```python
from build123d import *

# Parameters (mm, degrees)
SKETCH1_W           = 83
SKETCH1_H           = 126.35
SKETCH1_W_2         = 57.38
SKETCH1_H_2         = 90.25
BOSS_EXTRUDE1_DEPTH = 2
SKETCH2_W           = 78.4
SKETCH2_H           = 121.75
SKETCH2_W_2         = 76.4
SKETCH2_H_2         = 119.75
BOSS_EXTRUDE2_DEPTH = 1.5
FILLET1_R           = 3


with BuildPart() as part:
    # Sketch1 → Boss-Extrude1 (new body)
    with BuildSketch(Plane(origin=(0, 0, 0), x_dir=(1, 0, 0), z_dir=(0, 1, 0))):
        Rectangle(SKETCH1_W, SKETCH1_H)
        with Locations((0, 10.75)):
            Rectangle(SKETCH1_W_2, SKETCH1_H_2, mode=Mode.SUBTRACT)
    extrude(amount=BOSS_EXTRUDE1_DEPTH)

    # Sketch2 → Boss-Extrude2 (add)
    with BuildSketch(Plane(origin=(0, 2, 0), x_dir=(1, 0, 0), z_dir=(0, 1, 0))):
        Rectangle(SKETCH2_W, SKETCH2_H)
        Rectangle(SKETCH2_W_2, SKETCH2_H_2, mode=Mode.SUBTRACT)
    extrude(amount=BOSS_EXTRUDE2_DEPTH)

    # Fillet1
    fillet1_edges = [part.edges().sort_by_distance(p)[0] for p in [
        (-41.5, 1, -63.175),
        (41.5, 1, -63.175),
        (41.5, 1, 63.175),
        (-41.5, 1, 63.175),
    ]]
    fillet(fillet1_edges, radius=FILLET1_R)


solid = part.part
```
For this review, take the finished solid that the model builds, in its own axes (mm). Round coordinates to 2 decimals unless told otherwise and drop trailing zeros. Write each loop counter-clockwise with the first axis right and the second up, starting at its lowest first coordinate (ties: lowest second). Pieces come first, ordered by that corner, then holes. Notation, with made-up numbers: (-10.5, -40) -> (-6.5, -40) arc R23 ccw to (-6.5, -17) -> close; hole circle Ø3 at (12, 2.25). An arc over 180 degrees is marked (long way). Use one line per item in the form item = value.
1) Clearance check with flat-ended pins moving along their axes: pin 1 (8 mm diameter, centred on x = 25.5, z = 35.5, fed in from +Y); pin 2 (0.8 mm diameter, centred on x = -12.5, y = 2.5, fed in from +Z) (3 decimals); pin 3 (0.8 mm diameter, centred on y = 2.5, z = 16.5, fed in from +X). State where each tip first meets the part, or that it passes through.
Found:
pin_1 = 2
pin_2 = 60.875
pin_3 = 39.2
2) Take a section at A-A, the plane z = 23. Write out the cut boundary in (x, y), and give its area (3 significant figures).
Found:
outline = (-41.5, 0) -> (-28.69, 0) -> (-28.69, 2) -> (-38.2, 2) -> (-38.2, 3.5) -> (-39.2, 3.5) -> (-39.2, 2) -> (-41.5, 2) -> close; (28.69, 0) -> (41.5, 0) -> (41.5, 2) -> (39.2, 2) -> (39.2, 3.5) -> (38.2, 3.5) -> (38.2, 2) -> (28.69, 2) -> close
area = 54.2 mm2
3) Mouldability with a two-part tool opening along X and no side actions: class faces 1 (the flat face through (-40, 2, -19)), 2 (the cylindrical face through (40.6, 1.01, -62.32)), 3 (the flat face through (-1, 2, 39)), 4 (the cylindrical face through (-40.645, 1.014, 62.273)) as +X half, -X half, draft (parallel to the pull), parting line (faces both ways), or undercut.
Found:
face_1 = draft
face_2 = +X half
face_3 = undercut
face_4 = -X half
4) To check wall thickness, follow L1, parallel to Z at x = -29, y = 2.45 (3 decimals); L2, parallel to X at y = 2.15, z = -18; L3, parallel to Z at x = -3.5, y = 1 (3 decimals). State the ranges of each line that lie inside material, in increasing order. Write a range as from..to.
Found:
L1 = -60.875..-59.875, 59.875..60.875
L2 = -39.2..-38.2, 38.2..39.2
L3 = -63.175..-55.875, 34.375..63.175
5) Take a section at B-B, the plane x = -19. Write out the cut boundary in (y, z) (3 decimals).
Found:
outline = (0, -63.175) -> (2, -63.175) -> (2, -60.875) -> (3.5, -60.875) -> (3.5, -59.875) -> (2, -59.875) -> (2, -55.875) -> (0, -55.875) -> close; (0, 34.375) -> (2, 34.375) -> (2, 59.875) -> (3.5, 59.875) -> (3.5, 60.875) -> (2, 60.875) -> (2, 63.175) -> (0, 63.175) -> close
6) Take a section at C-C, the plane y = 2.85. Write out the cut boundary in (x, z) (3 decimals).
Found:
outline = (-39.2, -60.875) -> (39.2, -60.875) -> (39.2, 60.875) -> (-39.2, 60.875) -> close; hole (-38.2, -59.875) -> (38.2, -59.875) -> (38.2, 59.875) -> (-38.2, 59.875) -> close
7) Take a section at D-D, the plane z = 49. Write out the cut boundary in (x, y), and give its area (3 significant figures).
Found:
outline = (-41.5, 0) -> (41.5, 0) -> (41.5, 2) -> (39.2, 2) -> (39.2, 3.5) -> (38.2, 3.5) -> (38.2, 2) -> (-38.2, 2) -> (-38.2, 3.5) -> (-39.2, 3.5) -> (-39.2, 2) -> (-41.5, 2) -> close
area = 169 mm2
